Check sheet for the modelled part. Datum: model origin and axes. Units: mm. Face numbers are marked on the shaded views. A direction names the side the tool comes from. Coordinates: 2 decimals unless noted, no trailing zeros. Write each loop counter-clockwise with the first axis right and the second up, starting at its lowest first coordinate (ties: lowest second). Pieces come first, ordered by that corner, then holes. Notation, with made-up numbers: (20, -19.5) - (62, -19.5) arc R25 cw to (62, -5.5) - close; hole circle Ø1 at (-18.5, -13). An arc over 180 degrees is marked (long way). Write each question's results on one line, items separated by ' | '.
from build123d import *

# Parameters (mm, degrees)
SKETCH5_W           = 40
SKETCH5_H           = 10
BOSS_EXTRUDE4_DEPTH = 60
SKETCH11_W          = 15
SKETCH11_H          = 15
BOSS_EXTRUDE6_DEPTH = 10
FILLET1_R           = 6.5
SKETCH14_W          = 50
SKETCH14_H          = 15
BOSS_EXTRUDE7_DEPTH = 5
FILLET2_R           = 30
SKETCH16_R          = 6
BOSS_EXTRUDE8_DEPTH = 12
SKETCH17_W          = 64.115547938
SKETCH17_H          = 89.863494167
CUT_EXTRUDE1_DEPTH  = 2


with BuildPart() as part:
    # Sketch5 → Boss-Extrude4 (new body)
    with BuildSketch(Plane.XY):
        with Locations((-20, 5)):
            Rectangle(SKETCH5_W, SKETCH5_H)
    extrude(amount=BOSS_EXTRUDE4_DEPTH)

    # Sketch11 → Boss-Extrude6 (add)
    with BuildSketch(Plane(origin=(0, 10, 0), x_dir=(1, 0, 0), z_dir=(0, 1, 0))):
        with Locations((-20, -7.5)):
            Rectangle(SKETCH11_W, SKETCH11_H)
    extrude(amount=BOSS_EXTRUDE6_DEPTH)

    # Fillet1
    fillet1_edges = [part.edges().sort_by_distance(p)[0] for p in [
        (-27.5, 10, 7.5),
        (-20, 10, 15),
        (-12.5, 10, 7.5),
    ]]
    fillet(fillet1_edges, radius=FILLET1_R)

    # Sketch14 → Boss-Extrude7 (add)
    with BuildSketch(Plane.XY.offset(60)):
        with Locations((-20, 7.5)):
            Rectangle(SKETCH14_W, SKETCH14_H)
    extrude(amount=-BOSS_EXTRUDE7_DEPTH)

    # Fillet2
    # the kernel refuses this fillet: 30 mm, written as the material it adds along each edge
    with BuildSketch(Plane(origin=(0, 10, 55), x_dir=(0, 0, -1), z_dir=(0, -1, 0))) as fillet2_piece_1:
        with BuildLine():
            CenterArc((16.583123952, 30), FILLET2_R, 236.442690238, 33.557309762)
            Line((0, 5), (-0.331662479, 4.5))
            ThreePointArc((-0.331662479, 4.5), (-0.6, 2.5), (-0.6, 0))
            Line((-0.6, 0), (0, -0.6))
            Line((0, -0.6), (16.583123952, -0.6))
            Line((16.583123952, -0.6), (16.583123952, 0))
        make_face()
    extrude(amount=10)
    with BuildSketch(Plane(origin=(-40, 10, 55), x_dir=(0, 1, 0), z_dir=(1, 0, 0))) as fillet2_piece_2:
        with BuildLine():
            CenterArc((30, -16.583123952), FILLET2_R, 146.442690238, 33.557309762)
            Line((0, -16.583123952), (-0.6, -16.583123952))
            Line((-0.6, -16.583123952), (-0.6, 0))
            Line((-0.6, 0), (0, 0.6))
            ThreePointArc((0, 0.6), (2.5, 0.6), (4.5, 0.331662479))
            Line((4.5, 0.331662479), (5, 0))
        make_face()
    extrude(amount=40)
    with BuildSketch(Plane(origin=(-40, 0, 55), x_dir=(-1, 0, 0), z_dir=(0, 1, 0))) as fillet2_piece_3:
        with BuildLine():
            CenterArc((30, -16.583123952), FILLET2_R, 146.442690238, 33.557309762)
            Line((0, -16.583123952), (-0.6, -16.583123952))
            Line((-0.6, -16.583123952), (-0.6, 0))
            Line((-0.6, 0), (0, 0.6))
            ThreePointArc((0, 0.6), (2.5, 0.6), (4.5, 0.331662479))
            Line((4.5, 0.331662479), (5, 0))
        make_face()
    extrude(amount=10)
    with BuildSketch(Plane(origin=(0, 51.457809879, 55), x_dir=(0, 0, -1), z_dir=(0, -1, 0))) as fillet2_piece_4a_section:
        with BuildLine():
            CenterArc((16.583123952, 30), FILLET2_R, 236.442690238, 33.557309762)
            Line((0, 5), (-0.331662479, 4.5))
            ThreePointArc((-0.331662479, 4.5), (-0.6, 2.5), (-0.6, 0))
            Line((-0.6, 0), (0, -0.6))
            Line((0, -0.6), (16.583123952, -0.6))
            Line((16.583123952, -0.6), (16.583123952, 0))
        make_face()
    fillet2_piece_4a = extrude(amount=51.457809879, mode=Mode.PRIVATE)
    fillet2_piece_4a = split(fillet2_piece_4a, bisect_by=Plane(origin=(1.065152115, 10, 50.172088022), z_dir=(0, 1, 0)), keep=Keep.TOP, mode=Mode.PRIVATE)
    fillet2_piece_4a = split(fillet2_piece_4a, bisect_by=Plane(origin=(1.065152115, 15, 50.172088022), z_dir=(0, -1, 0)), keep=Keep.TOP, mode=Mode.PRIVATE)
    with BuildSketch(Plane(origin=(-40, 10, 55), x_dir=(0, 1, 0), z_dir=(1, 0, 0))) as fillet2_piece_4b_section:
        with BuildLine():
            CenterArc((30, -16.583123952), FILLET2_R, 146.442690238, 33.557309762)
            Line((0, -16.583123952), (-0.6, -16.583123952))
            Line((-0.6, -16.583123952), (-0.6, 0))
            Line((-0.6, 0), (0, 0.6))
            ThreePointArc((0, 0.6), (2.5, 0.6), (4.5, 0.331662479))
            Line((4.5, 0.331662479), (5, 0))
        make_face()
    fillet2_piece_4b = extrude(amount=81.457809879, mode=Mode.PRIVATE)
    fillet2_piece_4b = split(fillet2_piece_4b, bisect_by=Plane(origin=(0, 11.065152115, 50.172088022), z_dir=(1, 0, 0)), keep=Keep.TOP, mode=Mode.PRIVATE)
    fillet2_piece_4b = split(fillet2_piece_4b, bisect_by=Plane(origin=(5, 11.065152115, 50.172088022), z_dir=(-1, 0, 0)), keep=Keep.TOP, mode=Mode.PRIVATE)
    fillet2_piece_4 = fillet2_piece_4a & fillet2_piece_4b
    add(fillet2_piece_4)
    with BuildSketch(Plane(origin=(-81.457809879, 10, 55), x_dir=(0, 1, 0), z_dir=(1, 0, 0))) as fillet2_piece_5a_section:
        with BuildLine():
            CenterArc((30, -16.583123952), FILLET2_R, 146.442690238, 33.557309762)
            Line((0, -16.583123952), (-0.6, -16.583123952))
            Line((-0.6, -16.583123952), (-0.6, 0))
            Line((-0.6, 0), (0, 0.6))
            ThreePointArc((0, 0.6), (2.5, 0.6), (4.5, 0.331662479))
            Line((4.5, 0.331662479), (5, 0))
        make_face()
    fillet2_piece_5a = extrude(amount=81.457809879, mode=Mode.PRIVATE)
    fillet2_piece_5a = split(fillet2_piece_5a, bisect_by=Plane(origin=(-45, 11.065152115, 50.172088022), z_dir=(1, 0, 0)), keep=Keep.TOP, mode=Mode.PRIVATE)
    fillet2_piece_5a = split(fillet2_piece_5a, bisect_by=Plane(origin=(-40, 11.065152115, 50.172088022), z_dir=(-1, 0, 0)), keep=Keep.TOP, mode=Mode.PRIVATE)
    with BuildSketch(Plane(origin=(-40, 0, 55), x_dir=(-1, 0, 0), z_dir=(0, 1, 0))) as fillet2_piece_5b_section:
        with BuildLine():
            CenterArc((30, -16.583123952), FILLET2_R, 146.442690238, 33.557309762)
            Line((0, -16.583123952), (-0.6, -16.583123952))
            Line((-0.6, -16.583123952), (-0.6, 0))
            Line((-0.6, 0), (0, 0.6))
            ThreePointArc((0, 0.6), (2.5, 0.6), (4.5, 0.331662479))
            Line((4.5, 0.331662479), (5, 0))
        make_face()
    fillet2_piece_5b = extrude(amount=51.457809879, mode=Mode.PRIVATE)
    fillet2_piece_5b = split(fillet2_piece_5b, bisect_by=Plane(origin=(-41.065152115, 15, 50.172088022), z_dir=(0, -1, 0)), keep=Keep.TOP, mode=Mode.PRIVATE)
    fillet2_piece_5b = split(fillet2_piece_5b, bisect_by=Plane(origin=(-41.065152115, 10, 50.172088022), z_dir=(0, 1, 0)), keep=Keep.TOP, mode=Mode.PRIVATE)
    fillet2_piece_5 = fillet2_piece_5a & fillet2_piece_5b
    add(fillet2_piece_5)

    # Sketch16 → Boss-Extrude8 (add)
    with BuildSketch(Plane(origin=(0, 20, 0), x_dir=(1, 0, 0), z_dir=(0, 1, 0))):
        with Locations(Location((-20.072505657, -7.5, 0), (0, 0, 180))):
            Circle(SKETCH16_R)
    extrude(amount=BOSS_EXTRUDE8_DEPTH)

    # Sketch17 → Cut-Extrude1 (cut)
    with BuildSketch(Plane(origin=(0, 0, 0), x_dir=(-1, 0, 0), z_dir=(0, -1, 0))):
        with Locations((20.527974447, -24.438192458)):
            Rectangle(SKETCH17_W, SKETCH17_H)
    extrude(amount=-CUT_EXTRUDE1_DEPTH, mode=Mode.SUBTRACT)


solid = part.part
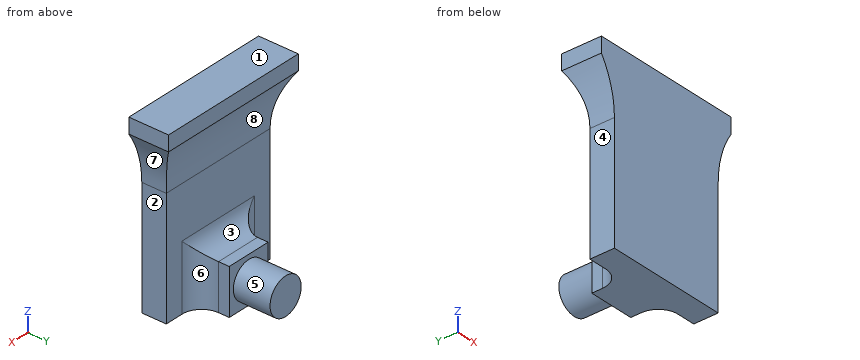
1. Access from +Z, -Z, +X, -X, +Y, -Y to the whole of each face (thin tool, end or side, straight path). Record for the marked faces 4, 5, 6, 7 and 8.
Values follow:
face 4: -Z, -X, +Y, -Y | face 5: +Y | face 6: -Z, +X, +Y | face 7: -Z, +X, +Y, -Y | face 8: +X, -X, +Y
2. Material ranges on L1, parallel to Y at x = -28.5, z = 32.5; L2, parallel to Z at x = -16, y = 16.25; L3, parallel to X at y = 19.5, z = 14, recorded low to high. Write a range as [from, to].
Values follow:
L1: y = [2, 10] | L2: z = [0, 15] | L3: x = [-27.5, -12.5]
3. Draft check along Z on the marked faces 1, 2 and 3. Enter one of: pulls with the +Z half, pulls with the -Z half, needs draft (parallel to the pull), parting line crosses it, or undercut.
Values follow:
face 1: pulls with the +Z half | face 2: needs draft | face 3: undercut
4. Sectioned sample at D-D (y = 21.5). Record the cut outline in (x, z), then the cut area to 3 significant figures.
Values follow:
outline: circle Ø12 at (-20.07, 7.5) | area: 113 mm^2
5. Sectioned sample at B-B (x = -31.5). Record the cut outline in (y, z).
Values follow:
outline: (2, 0) - (10.5, 0) - (10.5, 19) arc R6.5 cw to (10, 21.5) - (10, 38.42) arc R30 cw to (15, 55) - (15, 60) - (2, 60) - close
6. Sectioned sample at A-A (y = 14). Record the cut outline in (x, z), then the cut area to 3 significant figures.
Values follow:
outline: (-45, 55) arc R30 cw to (-44, 53.38) - (4, 53.38) arc R30 cw to (5, 55) - (5, 60) - (-45, 60) - close; (-28, 0) - (-12, 0) - (-12, 15.5) - (-28, 15.5) - close | area: 577 mm^2
7. Go/stop test with flat-tipped pins: pin 1 (3 mm diameter, centred on y = 10.5, z = 12, fed in from +X); pin 2 (8 mm diameter, centred on x = -35.5, z = 54, fed in from +Y); pin 3 (6.5 mm diameter, centred on y = 7, z = 23.5, fed in from -X). Record where each tip stops, or that it passes through.
Values follow:
pin 1: stops at x = 0 | pin 2: stops at y = 15 | pin 3: stops at x = -40
8. Sectioned sample at C-C (z = 7.5). Record the cut outline in (x, y).
Values follow:
outline: (-40, 2) - (0, 2) - (0, 10) - (-6, 10) arc R6.5 cw to (-12.5, 16.5) - (-12.5, 20) - (-14.07, 20) - (-14.07, 32) - (-26.07, 32) - (-26.07, 20) - (-27.5, 20) - (-27.5, 16.5) arc R6.5 cw to (-34, 10) - (-40, 10) - close
